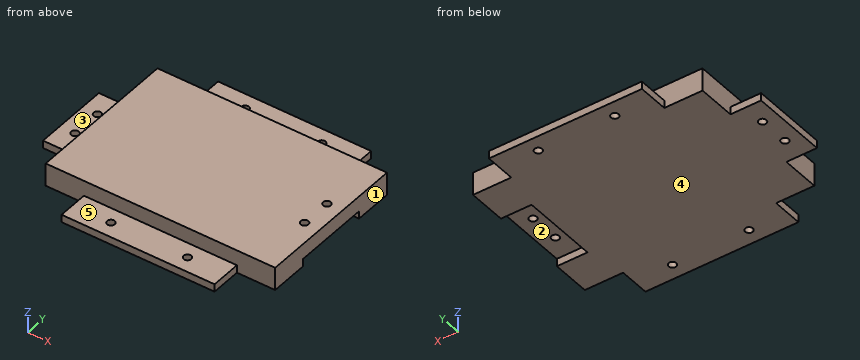
Autodesk Inventor part; units mm, degrees
ref_plane "YZ Plane" through (0, 0, 0) normal (1, 0, 0) x (0, 1, 0)
ref_plane "XZ Plane" through (0, 0, 0) normal (0, 1, 0) x (-1, 0, 0)
ref_plane "XY Plane" through (0, 0, 0) normal (0, 0, 1) x (1, 0, 0)
sketch "Sketch1" plane through (0, 0, 0) normal (0, 0, 1) x (1, 0, 0)
  line L0 (0, 0) -> (150, 0)
  line L1 (150, 0) -> (150, 100)
  line L2 (150, 100) -> (0, 100)
  line L3 (0, 100) -> (0, 0)
  dimension "d0" = 150
  dimension "d1" = 100
extrude "Extrusion1" add sketch "Sketch1" along normal blind 15
sketch "Sketch7" plane through (0, 0, 0) normal (0, 0, -1) x (-1, 0, 0)
  line L0 (0, 25) -> (20, 25)
  line L1 (20, 25) -> (20, 75)
  line L2 (20, 75) -> (0, 75)
  line L3 (0, 75) -> (0, 25)
  point P0 (0, 0)
  dimension "d27" = 20
  dimension "d28" = 50
  dimension "d29" = 25
extrude "Extrusion7" add sketch "Sketch7" against normal blind 5
sketch "Sketch8" plane through (0, 0, 0) normal (0, 0, -1) x (-1, 0, 0)
  line L0 (-25, 0) -> (-125, 0)
  line L1 (-125, 0) -> (-125, -20)
  line L2 (-125, -20) -> (-25, -20)
  line L3 (-25, -20) -> (-25, 0)
  line L4 (-150, 100) -> (0, 100)
  line L5 (-25, 100) -> (-125, 100)
  line L6 (-125, 100) -> (-125, 120)
  line L7 (-125, 120) -> (-25, 120)
  line L8 (-25, 120) -> (-25, 100)
  point P0 (0, 0)
  dimension "d32" = 100
  dimension "d33" = 20
  dimension "d34" = 25
  dimension "d37" = 100
  dimension "d38" = 20
extrude "Extrusion8" add sketch "Sketch8" against normal blind 5
sketch "Sketch9" plane through (0, 0, 0) normal (0, 0, -1) x (-1, 0, 0)
  circle A0 centre (-50, -10) radius 2.5
  circle A1 centre (-100, -10) radius 2.5
  line L0 (-25, -20) -> (-25, 0)
  line L1 (-125, 0) -> (-125, -20)
  line L2 (-25, 0) -> (-125, 0)
  circle A2 centre (-50, 110) radius 2.5
  circle A3 centre (-100, 110) radius 2.5
  line L3 (-125, 120) -> (-25, 120)
  circle A4 centre (10, 40) radius 2.5
  circle A5 centre (10, 60) radius 2.5
  line L4 (0, 75) -> (0, 25)
  line L5 (0, 25) -> (20, 25)
  line L6 (20, 75) -> (0, 75)
  point P0 (0, 0)
  dimension "d39" = 5
  dimension "d40" = 5
  dimension "d41" = 25
  dimension "d42" = 25
  dimension "d43" = 10
  dimension "d44" = 5
  dimension "d45" = 5
  dimension "d46" = 10
  dimension "d47" = 5
  dimension "d48" = 5
  dimension "d49" = 10
  dimension "d50" = 15
  dimension "d51" = 15
extrude "Extrusion9" cut sketch "Sketch9" against normal through all
thread "Thread1"
thread "Thread2"
thread "Thread3"
thread "Thread4"
thread "Thread5"
thread "Thread6"
sketch "Sketch10" plane through (0, 0, 0) normal (0, 0, -1) x (-1, 0, 0)
  line L0 (-150, 0) -> (-150, 100)
  line L1 (-150, 25) -> (-130, 25)
  line L2 (-130, 25) -> (-130, 75)
  line L3 (-130, 75) -> (-150, 75)
  line L4 (-150, 75) -> (-150, 25)
  circle A0 centre (10, 40) radius 2.5
  circle A1 centre (-50, 110) radius 2.5
  circle A2 centre (-50, -10) radius 2.5
  circle A3 centre (-100, -10) radius 2.5
  circle A4 centre (-100, 110) radius 2.5
  circle A5 centre (10, 60) radius 2.5
  line L5 (0, 0) -> (-25, 0)
  line L6 (0, 25) -> (0, 0)
  line L7 (0, 25) -> (20, 25)
  line L8 (20, 25) -> (20, 75)
  line L9 (20, 75) -> (0, 75)
  line L10 (0, 100) -> (0, 75)
  line L11 (-25, 100) -> (0, 100)
  line L12 (-25, 120) -> (-25, 100)
  line L13 (-125, 120) -> (-25, 120)
  line L14 (-125, 100) -> (-125, 120)
  line L15 (-150, 100) -> (-125, 100)
  line L16 (-150, 0) -> (-150, 100)
  line L17 (-125, 0) -> (-150, 0)
  line L18 (-125, 0) -> (-125, -20)
  line L19 (-125, -20) -> (-25, -20)
  line L20 (-25, -20) -> (-25, 0)
  dimension "d66" = 20
  dimension "d67" = 50
extrude "Extrusion10" cut sketch "Sketch10" against normal blind 5 contours L0 L3 L2 L1
sketch "Sketch11" plane through (0, 0, 5) normal (0, 0, -1) x (-1, 0, 0)
  circle A0 centre (-140, 60) radius 2.5
  circle A1 centre (-140, 40) radius 2.5
  line L0 (-130, 25) -> (-150, 25)
  line L1 (-150, 0) -> (-150, 25)
  line L2 (-125, 0) -> (-150, 0)
  line L3 (-125, 0) -> (-125, -20)
  line L4 (-125, -20) -> (-25, -20)
  line L5 (-25, -20) -> (-25, 0)
  line L6 (0, 0) -> (-25, 0)
  line L7 (0, 25) -> (0, 0)
  line L8 (0, 25) -> (20, 25)
  line L9 (20, 25) -> (20, 75)
  line L10 (20, 75) -> (0, 75)
  line L11 (0, 100) -> (0, 75)
  line L12 (-25, 100) -> (0, 100)
  line L13 (-25, 120) -> (-25, 100)
  line L14 (-125, 120) -> (-25, 120)
  line L15 (-125, 100) -> (-125, 120)
  line L16 (-150, 100) -> (-125, 100)
  line L17 (-150, 75) -> (-150, 100)
  line L18 (-150, 75) -> (-130, 75)
  line L19 (-130, 75) -> (-130, 25)
  circle A2 centre (10, 40) radius 2.5
  circle A3 centre (-50, 110) radius 2.5
  circle A4 centre (-50, -10) radius 2.5
  circle A5 centre (-100, -10) radius 2.5
  circle A6 centre (-100, 110) radius 2.5
  circle A7 centre (10, 60) radius 2.5
  line L20 (-150, 25) -> (-150, 75)
  dimension "d70" = 5
  dimension "d71" = 5
  dimension "d72" = 10
  dimension "d79" = 15
extrude "Extrusion11" cut sketch "Sketch11" against normal through all contours A0 | A1
thread "Thread7"
thread "Thread8"
properties part number "CP007" material "ABS Plastic"
For this review, take the finished solid that the model builds, in its own axes (mm). Face numbers are marked on the shaded views. A direction names the side the tool comes from. Give positions to 0.01 mm unless a question says otherwise; leave off trailing zeros. Write each loop counter-clockwise with the first axis right and the second up, starting at its lowest first coordinate (ties: lowest second). Pieces come first, ordered by that corner, then holes.
Item 1: Take a section at C-C (z = 2.5). Give the boundary of the cut face in (x, y).
Item 2: Take a section at A-A (x = -10). Give the boundary of the cut face in (y, z).
Item 3: Take a section at B-B (y = 110). Give the boundary of the cut face in (x, z), and give its area (3 significant figures).
Item 4: Take a section at D-D (x = 140). Give the boundary of the cut face in (y, z).
Item 5: Machinability: for the marked faces 3, 4 and 5, which of the approach directions +Z, -Z, +X, -X, +Y, -Y give a long, thin tool a straight path to every point of the face, cutting with its end or side? Answer none if there is none.
Item 6: The part is to be moulded in two halves that separate along Y. For the marked faces 1 and 2, say which applies: +Y half, -Y half, draft (parallel to the pull), parting line (faces both ways), or undercut.
Item 7: Insertion check: P1, Ø6, axis at x = 28.5, z = 10, coming from the +Y side; P2, Ø1, axis at y = 32.5, z = 2.5, coming from the +X side; P3, Ø22, axis at x = 56, y = -12.5, coming from the +Z side. Each pin has a flat end and moves straight along its axis. Give the tip position at first contact, or say it passes through.
Item 8: Wall thickness on probe 1 along Y at (x, z) = (100, 3.85); probe 2 along Y at (x, z) = (140, 11.5); probe 3 along X at (y, z) = (28, 8): over which ranges is each line inside the solid? List them lowest first.
Established:
1. outline: (-20, 25) - (0, 25) - (0, 0) - (25, 0) - (25, -20) - (125, -20) - (125, 0) - (150, 0) - (150, 25) - (130, 25) - (130, 75) - (150, 75) - (150, 100) - (125, 100) - (125, 120) - (25, 120) - (25, 100) - (0, 100) - (0, 75) - (-20, 75) - close; hole circle Ø5 at (-10, 40); hole circle Ø5 at (-10, 60); hole circle Ø5 at (50, -10); hole circle Ø5 at (50, 110); hole circle Ø5 at (100, -10); hole circle Ø5 at (100, 110)
2. outline: (25, 0) - (37.5, 0) - (37.5, 5) - (25, 5) - close; (42.5, 0) - (57.5, 0) - (57.5, 5) - (42.5, 5) - close; (62.5, 0) - (75, 0) - (75, 5) - (62.5, 5) - close
3. outline: (25, 0) - (47.5, 0) - (47.5, 5) - (25, 5) - close; (52.5, 0) - (97.5, 0) - (97.5, 5) - (52.5, 5) - close; (102.5, 0) - (125, 0) - (125, 5) - (102.5, 5) - close
3. area: 450 mm2
4. outline: (0, 0) - (25, 0) - (25, 5) - (37.5, 5) - (37.5, 15) - (0, 15) - close; (42.5, 5) - (57.5, 5) - (57.5, 15) - (42.5, 15) - close; (62.5, 5) - (75, 5) - (75, 0) - (100, 0) - (100, 15) - (62.5, 15) - close
5. face 3: +Z, -X, +Y, -Y
5. face 4: -Z, +X, -X, +Y, -Y
5. face 5: +Z, +X, -X, -Y
6. face 1: draft
6. face 2: undercut
7. P1: stops at y = 100
7. P2: stops at x = 130
7. P3: stops at z = 5
8. probe 1: y = -20 to -12.5, -7.5 to 107.5, 112.5 to 120
8. probe 2: y = 0 to 37.5, 42.5 to 57.5, 62.5 to 100
8. probe 3: x = 0 to 150
